CAD build for the part. Positions are in the model's coordinates, mm. A direction names the side the tool comes from. Give positions to 0.01 mm unless a question says otherwise; leave off trailing zeros. Write each loop counter-clockwise with the first axis right and the second up, starting at its lowest first coordinate (ties: lowest second). Pieces come first, ordered by that corner, then holes. Notation, with made-up numbers: (29, -28.5) - (44, -28.5) arc R10 ccw to (44, -11.5) - close; hole circle Ø10 at (39.25, 45.25). An arc over 180 degrees is marked (long way). Put each result on its own line as item: value. Start each with the question number.
1. Cut at A-A on x = -3.5. List the corners of the cut face in (y, z).
2. Tool access for faces 1 (the flat face through (0, 0, 0)), 2 (the flat face through (-3, 18.1, 0)), 3 (the flat face through (4.1, 2, 0)), 4 (the flat face through (6.1, 1, 0)): list every direction of +Z, -Z, +X, -X, +Y, -Y with a clear straight run to the whole face (end or side of a thin tool).
3. Cut at B-B on y = 1.25. List the corners of the cut face in (x, z), and give its area (3 significant figures).
4. Drop flat-ended pins along their axis: pin 1 (6 mm diameter, centred on y = 2, z = -11, fed in from +X); pin 2 (3 mm diameter, centred on y = 10.5, z = -8, fed in from -X); pin 3 (4.5 mm diameter, centred on y = 0.5, z = 1, fed in from +X). Give the stop position or say it passes through.
5. Cut at D-D on x = -0.25. List the corners of the cut face in (y, z).
6. Wall check: line 1 (Y direction, x = -3.5, z = 6.5); line 2 (X direction, y = 1.5, z = 7.25); line 3 (X direction, y = 17.5, z = 11). Give the ranges that are in metal, low to high.
7. Mould opens along Y. For faces 5 (the flat face through (5, 3.5, 0)), 6 (the flat face through (-4.1, 9, 0)), 7 (the flat face through (-6.1, 9, 0)) say: +Y half, -Y half, draft (parallel to the pull), parting line (faces both ways), or undercut.
8. Cut at C-C on z = -8.5. List the corners of the cut face in (x, y), and give its area (4 significant figures).
Autodesk Inventor part; units mm, degrees
ref_plane "YZ Plane" through (0, 0, 0) normal (1, 0, 0) x (0, 1, 0)
ref_plane "XZ Plane" through (0, 0, 0) normal (0, 1, 0) x (-1, 0, 0)
ref_plane "XY Plane" through (0, 0, 0) normal (0, 0, 1) x (1, 0, 0)
sketch "Skizze1" plane through (0, 0, 0) normal (0, 1, 0) x (-1, 0, 0)
  line L0 (4.1, 15) -> (-4.1, 15)
  line L1 (-4.1, 15) -> (-4.1, -15)
  line L2 (-4.1, -15) -> (4.1, -15)
  line L3 (4.1, -15) -> (4.1, 15)
  line L4 (4.1, 15) -> (-4.1, -15) construction
  line L5 (-4.1, 15) -> (4.1, -15) construction
  line L6 (6.1, 17) -> (-6.1, 17)
  line L7 (-6.1, 17) -> (-6.1, -17)
  line L8 (-6.1, -17) -> (6.1, -17)
  line L9 (6.1, -17) -> (6.1, 17)
  line L10 (6.1, 17) -> (-6.1, -17) construction
  line L11 (-6.1, 17) -> (6.1, -17) construction
  point P0 (0, 0)
  dimension "d0" = 8.2
  dimension "d1" = 30
  dimension "d2" = 12.2
  dimension "d3" = 34
extrude "Extrusion1" add sketch "Skizze1" along normal blind 18.1
sketch "Skizze2" plane through (0, 0, 0) normal (0, -1, 0) x (1, 0, 0)
  line L0 (6.1, 17) -> (6.1, -17)
  line L1 (-6.1, 17) -> (6.1, 17)
  line L2 (-6.1, -17) -> (-6.1, 17)
  line L3 (6.1, -17) -> (-6.1, -17)
  line L4 (-4.1, 15) -> (-4.1, -15)
  line L5 (4.1, 15) -> (-4.1, 15)
  line L6 (4.1, -15) -> (4.1, 15)
  line L7 (-4.1, -15) -> (4.1, -15)
  point P0 (0, 0)
extrude "Extrusion2" add sketch "Skizze2" along normal blind 2 contours L0 L3 L2 L1 | L5 L6 L7 L4
sketch "Skizze3" plane through (6.1, 18.1, 17) normal (1, 0, 0) x (0, 0, -1)
  line L0 (2, -18.1) -> (32, -18.1)
  line L1 (32, -18.1) -> (32, 0)
  line L2 (2, 0) -> (32, 0)
  line L3 (2, -18.1) -> (2, 0)
  line L4 (32, -18.1) -> (32, 0)
  line L5 (2, -18.1) -> (32, -18.1)
  line L6 (32, -18.1) -> (32, -14.6)
  line L7 (32, -14.6) -> (2, -14.6)
  line L8 (2, -14.6) -> (2, -18.1)
  point P0 (17, -18.1)
  point P1 (2, -14.6)
  dimension "d8" = 3.5
extrude "Extrusion3" cut sketch "Skizze3" against normal up to surface (2 mm away) contours L3 L2 L1 L7
sketch "Skizze4" plane through (0, 18.1, 0) normal (0, 1, 0) x (1, 0, 0)
  line L0 (-4.1, -15) -> (-4.1, 15)
  line L1 (4.1, -15) -> (-4.1, -15)
  line L2 (-4.1, 15) -> (-3.5, 15)
  line L3 (-3.5, 15) -> (-3.5, -15)
  line L4 (-3.5, -15) -> (-4.1, -15)
  line L5 (-4.1, -15) -> (-4.1, 15)
  line L6 (-3.5, 15) -> (-2.9, 15)
  line L7 (-2.9, 15) -> (-2.9, -15)
  line L8 (-2.9, -15) -> (-3.5, -15)
  line L9 (-3.5, -15) -> (-3.5, 15)
  line L10 (-6.1, 17) -> (6.1, 17)
  line L11 (-6.1, -17) -> (6.1, -17)
  line L12 (-6.1, 17) -> (-2.9, 17)
  line L13 (-2.9, 17) -> (-2.9, -17)
  line L14 (-2.9, -17) -> (-6.1, -17)
  line L15 (-6.1, -17) -> (-6.1, 17)
  point P0 (0, 0)
  dimension "d11" = 0.6
  dimension "d12" = 0.6
extrude "Extrusion4" add sketch "Skizze4" along normal blind 1
sketch "Skizze6" plane through (-4.1, 0, -15) normal (0, 0, 1) x (1, 0, 0)
  line L0 (10.2, -2) -> (10.2, 18.1)
  line L1 (0, 0) -> (0, 18.1)
  line L2 (10.2, 18.1) -> (0, 18.1)
  line L3 (0, 18.1) -> (0, 3.5)
  line L4 (0, 3.5) -> (10.2, 3.5)
  line L5 (10.2, 3.5) -> (10.2, 18.1)
  point P0 (4.1, 0)
  dimension "d30" = 14.6
extrude "Extrusion6" cut sketch "Skizze6" against normal through all
mirror "Spiegeln1" about plane through (0, 0, 0) normal (0, 0, 1) of "Extrusion6"
sketch "Skizze7" plane through (-4.1, 0, -15) normal (0, 0, 1) x (1, 0, 0)
  line L0 (8.2, 3.5) -> (0, 3.5)
  line L1 (0, 0) -> (0, 3.5)
  line L2 (0, 0) -> (8.2, 0)
  line L3 (8.2, 0) -> (8.2, 3.5)
  point P0 (4.1, 0)
extrude "Extrusion7" cut sketch "Skizze7" along normal through all both and the other way through all
sketch "Skizze8" plane through (6.1, -2, -17) normal (0, 0, -1) x (-1, 0, 0)
  line L0 (2, 2) -> (2, 5.5)
  line L1 (2, 5.5) -> (0, 5.5)
  line L2 (0, 0) -> (0, 5.5)
  line L3 (12.2, 0) -> (0, 0)
  line L4 (12.2, 0) -> (12.2, 21.1)
  line L5 (9, 21.1) -> (12.2, 21.1)
  line L6 (9, 20.1) -> (9, 21.1)
  line L7 (9, 20.1) -> (10.2, 20.1)
  line L8 (10.2, 20.1) -> (10.2, 2)
  line L9 (10.2, 2) -> (2, 2)
  point P0 (6.1, 2)
extrude "Extrusion8" cut sketch "Skizze8" against normal blind 2
mirror "Spiegeln2" about plane through (0, 0, 0) normal (0, 0, 1) of "Extrusion8"
sketch "Skizze10" plane through (-6.1, -2, 15) normal (0, 0, 1) x (1, 0, 0)
  line L0 (12.2, 0) -> (0, 0)
  line L1 (0, 0) -> (-1.5, 0)
  line L2 (-1.5, 0) -> (-1.5, 1.5)
  line L3 (-1.5, 1.5) -> (0, 1.5)
  line L4 (0, 1.5) -> (0, 0)
  line L5 (12.2, 0) -> (13.7, 0)
  line L6 (13.7, 0) -> (13.7, 1.5)
  line L7 (13.7, 1.5) -> (12.2, 1.5)
  line L8 (12.2, 1.5) -> (12.2, 0)
  line L9 (0, 1.5) -> (-1.5, 0)
  line L10 (12.2, 1.5) -> (13.7, 0)
  point P0 (6.1, 2)
  dimension "d44" = 1.5
  dimension "d45" = 1.5
  dimension "d46" = 1.5
  dimension "d47" = 1.5
extrude "Extrusion10" add sketch "Skizze10" against normal up to surface (30 mm away) contours L1 L9 L4 | L8 L10 L5
sketch "Skizze11" plane through (-2.9, 18.1, -15) normal (1, 0, 0) x (0, 0, -1)
  line L0 (-30, 1) -> (-30, 0)
  line L1 (0, 0) -> (-30, 0)
  line L2 (0, 0) -> (0, 1)
  line L3 (-30, 1) -> (0, 1)
  point P0 (-15, -18.1)
extrude "Extrusion11" add sketch "Skizze11" along normal blind 0.4
properties part number "WagoHolder"
Report:
1. outline: (-2, -15) - (0, -15) - (0, 15) - (-2, 15) - close; (18.1, -15) - (19.1, -15) - (19.1, 15) - (18.1, 15) - close
2. face 1: +Z, -Z
2. face 2: +Z, -Z, +X
2. face 3: +Z, -Z, +Y
2. face 4: +Z, -Z, +X, +Y
3. outline: (-6.1, -15) - (-4.1, -15) - (-4.1, 15) - (-6.1, 15) - close; (4.1, -15) - (6.1, -15) - (6.1, 15) - (4.1, 15) - close
3. area: 120 mm²
4. pin 1: stops at x = 6.6
4. pin 2: stops at x = -6.1
4. pin 3: stops at x = 7.35
5. outline: (-2, -15) - (0, -15) - (0, 15) - (-2, 15) - close
6. line 1: y = -2 to 0, 18.1 to 19.1
6. line 2: x = -6.1 to -4.1, 4.1 to 6.1
6. line 3: x = -6.1 to -4.1
7. face 5: +Y half
7. face 6: undercut
7. face 7: draft
8. outline: (-7.6, -2) - (7.6, -2) - (6.1, -0.5) - (6.1, 3.5) - (4.1, 3.5) - (4.1, 0) - (-4.1, 0) - (-4.1, 18.1) - (-2.5, 18.1) - (-2.5, 19.1) - (-6.1, 19.1) - (-6.1, -0.5) - close
8. area: 73.45 mm²
